The drawing under review shows one solid part. Ordinate dimensions are in mm from its lowest x, y, z. Give positions to 0.01 mm unless a question says otherwise; leave off trailing zeros. Order: outer loops, then holes, each group sorted by start corner. A loop starts at its lowest first (then second) coordinate and runs counter-clockwise, first axis right, second up. Notation, with made-up numbers: M -20.5,40 L 37.5,40 A15 ccw 37.5,53 Z; hole C 29.25,-5.5 d4. An arc over 180 degrees is marked long. Put each result on its own line as item: value. Start each with the question number.
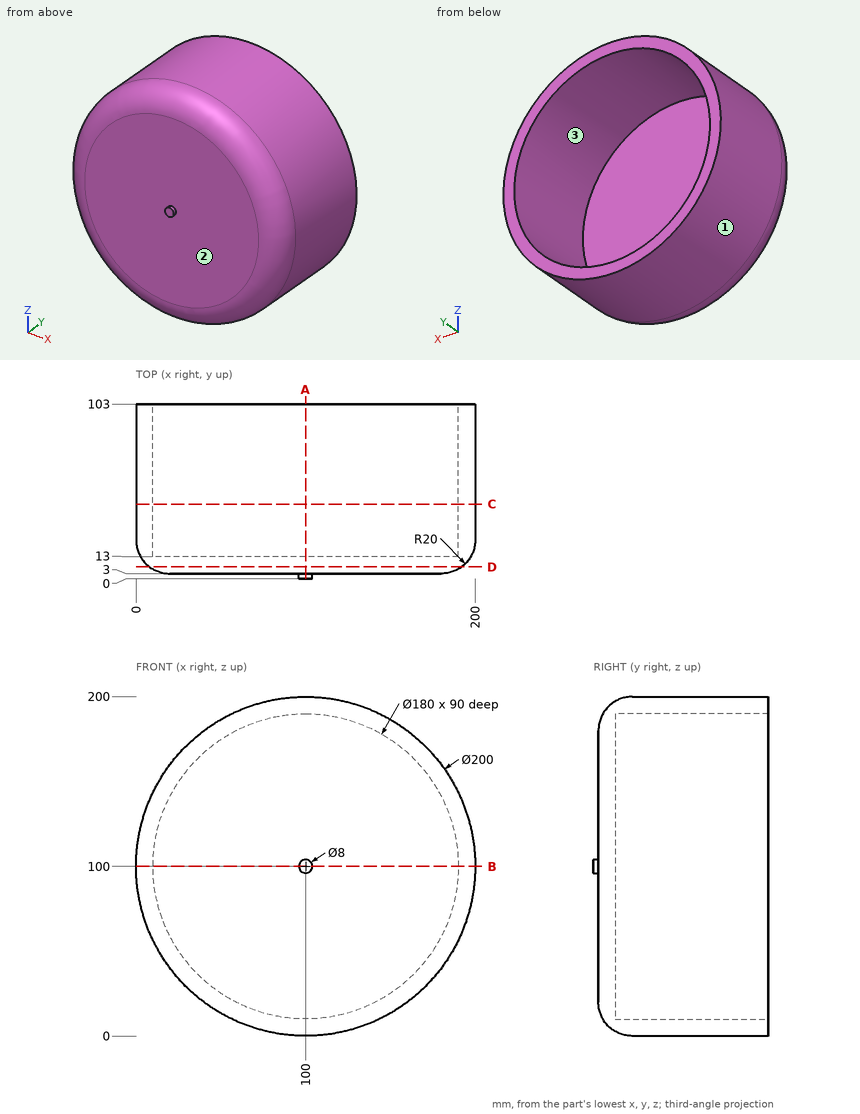
1. The part is to be moulded in two halves that separate along X. For the marked faces 1, 2 and 3, say which applies: +X half, -X half, draft (parallel to the pull), parting line (faces both ways), or undercut.
2. Consider section B-B on z = 100. Give the boundary of the cut face in (x, y), then the cut area to 3 significant figures.
3. Consider section D-D on y = 7. Give the boundary of the cut face in (x, z).
4. Consider section C-C on y = 44. Give the boundary of the cut face in (x, z), then the cut area to 3 significant figures.
5. Insertion check: pin 1 (1 mm diameter, centred on x = 114, z = 21, fed in from +Y); pin 2 (2 mm diameter, centred on y = 19.5, z = 58.5, fed in from -X); pin 3 (1 mm diameter, centred on y = 53.5, z = 54, fed in from +X). Each pin has a flat end and moves straight along its axis. Give the tip position at first contact, or say it passes through.
6. To check wall thickness, follow probe 1 along X at (y, z) = (77, 100); probe 2 along X at (y, z) = (36, 108); probe 3 along Y at (x, z) = (59, 70). State the ranges of each line that lie inside material, in increasing order.
7. Consider section A-A on x = 100. Give the boundary of the cut face in (y, z), then the cut area to 3 significant figures.
Returned:
1. face 1: parting line
1. face 2: draft
1. face 3: undercut
2. outline: M 0,23 A20 ccw 20,3 L 96,3 L 96,0 L 104,0 L 104,3 L 180,3 A20 ccw 200,23 L 200,103 L 190,103 L 190,13 L 10,13 L 10,103 L 0,103 Z
2. area: 3,650 mm2
3. outline: C 100,100 d184
4. outline: C 100,100 d200; hole C 100,100 d180
4. area: 5,970 mm2
5. pin 1: stops at y = 13
5. pin 2: stops at x = 8.87
5. pin 3: stops at x = 189.05
6. probe 1: x = 0 to 10, 190 to 200
6. probe 2: x = 0.32 to 10.36, 189.64 to 199.68
6. probe 3: y = 3 to 13
7. outline: M 0,96 L 3,96 L 3,20 A20 ccw 23,0 L 103,0 L 103,10 L 13,10 L 13,190 L 103,190 L 103,200 L 23,200 A20 ccw 3,180 L 3,104 L 0,104 Z
7. area: 3,650 mm2
